```python
from build123d import *

# Parameters (mm, degrees)
BOSS_EXTRUDE1_DEPTH = 6.5
FILLET1_R           = 3


with BuildPart() as part:
    # Sketch1 → Boss-Extrude1 (new body)
    with BuildSketch(Plane(origin=(0, 0, 0), x_dir=(1, 0, 0), z_dir=(0, 1, 0))):
        Polygon((0, 0), (16, 0), (26.5, 0), (26.5, 10), (16, 10), (16, 30), (0, 30), (0, 10), (-10.5, 10), (-10.5, 0), align=None)
    extrude(amount=BOSS_EXTRUDE1_DEPTH)

    # Fillet1
    fillet1_edges = [part.edges().sort_by_distance(p)[0] for p in [
        (0, 3.25, -10),
        (0, 3.25, -30),
        (16, 3.25, -30),
        (16, 3.25, -10),
        (26.5, 3.25, -10),
        (-10.5, 3.25, -10),
    ]]
    fillet(fillet1_edges, radius=FILLET1_R)


solid = part.part
```
Verification items for the finished model (mm, model axes). A direction names the side the tool comes from. Coordinates: 2 decimals unless noted, no trailing zeros. Loops run counter-clockwise (first coordinate to the right, second up) from the corner with the lowest first, then second, coordinate; pieces in that order, holes last. Notation, with made-up numbers: (44, 15.5) - (60, 15.5) arc R23 ccw to (60, 30.5) - close; hole circle Ø11 at (49.5, 20.5). An arc over 180 degrees is marked (long way). Return JSON: item names as keys, results as strings.
1. Section check A-A, the plane y = 1.5. Record the boundary of the cut face in (x, z), then the cut area to 3 significant figures.
Established:
{"outline": "(-10.5, -7) arc R3 ccw to (-7.5, -10) - (-3, -10) arc R3 cw to (0, -13) - (0, -27) arc R3 ccw to (3, -30) - (13, -30) arc R3 ccw to (16, -27) - (16, -13) arc R3 cw to (19, -10) - (23.5, -10) arc R3 ccw to (26.5, -7) - (26.5, 0) - (-10.5, 0) - close", "area": "686 mm2"}
2. Tool access check on faces 1 (the flat face through (26.5, 3, -3)), 2 (the flat face through (-5, 3, -10)), 3 (the flat face through (16, 3, -20)). Record the directions out of +Z, -Z, +X, -X, +Y, -Y that give a thin tool (end or side, any length) a straight path to the whole face; none if there is none.
Established:
{"face 1": "+Z, -Z, +X, +Y, -Y", "face 2": "-Z, -X, +Y, -Y", "face 3": "-Z, +X, +Y, -Y"}
3. Thickness scan on L1, parallel to X at y = 5.25, z = -20.5; L2, parallel to Z at x = -7, y = 1.5; L3, parallel to Z at x = -0.5, y = 3.5. Record the ranges inside material, lowest first.
Established:
{"L1": "x = 0 to 16", "L2": "z = -10 to 0", "L3": "z = -11.34 to 0"}
4. Go/stop test with flat-tipped pins: pin 1 (12 mm diameter, centred on x = -6.5, z = -19, fed in from -Y) (1 decimal); pin 2 (1.3 mm diameter, centred on x = -6.5, y = 3, fed in from -Z); pin 3 (1.5 mm diameter, centred on y = 1.5, z = -15, fed in from +X). Record where each tip stops, or that it passes through.
Established:
{"pin 1": "passes through", "pin 2": "stops at z = -10", "pin 3": "stops at x = 16"}
5. Section check B-B, the plane x = -3.5. Record the boundary of the cut face in (y, z), then the cut area to 3 significant figures.
Established:
{"outline": "(0, -10) - (6.5, -10) - (6.5, 0) - (0, 0) - close", "area": "65.0 mm2"}
6. Section check C-C, the plane z = -17.5. Record the boundary of the cut face in (x, y), then the cut area to 3 significant figures.
Established:
{"outline": "(0, 0) - (16, 0) - (16, 6.5) - (0, 6.5) - close", "area": "104 mm2"}
